Could you check a few things on this drawing? It's one solid part, dimensions in mm from its lowest x, y, z. A direction names the side the tool comes from. Round coordinates to 2 decimals unless told otherwise and drop trailing zeros. Loops run counter-clockwise (first coordinate to the right, second up) from the corner with the lowest first, then second, coordinate; pieces in that order, holes last. Notation, with made-up numbers: M 57.25,69.5 L 65.25,69.5 A32 ccw 65.25,104.5 Z; hole C -5,36 d10. An arc over 180 degrees is marked long. Write item = value, one per line. Start each with the question number.
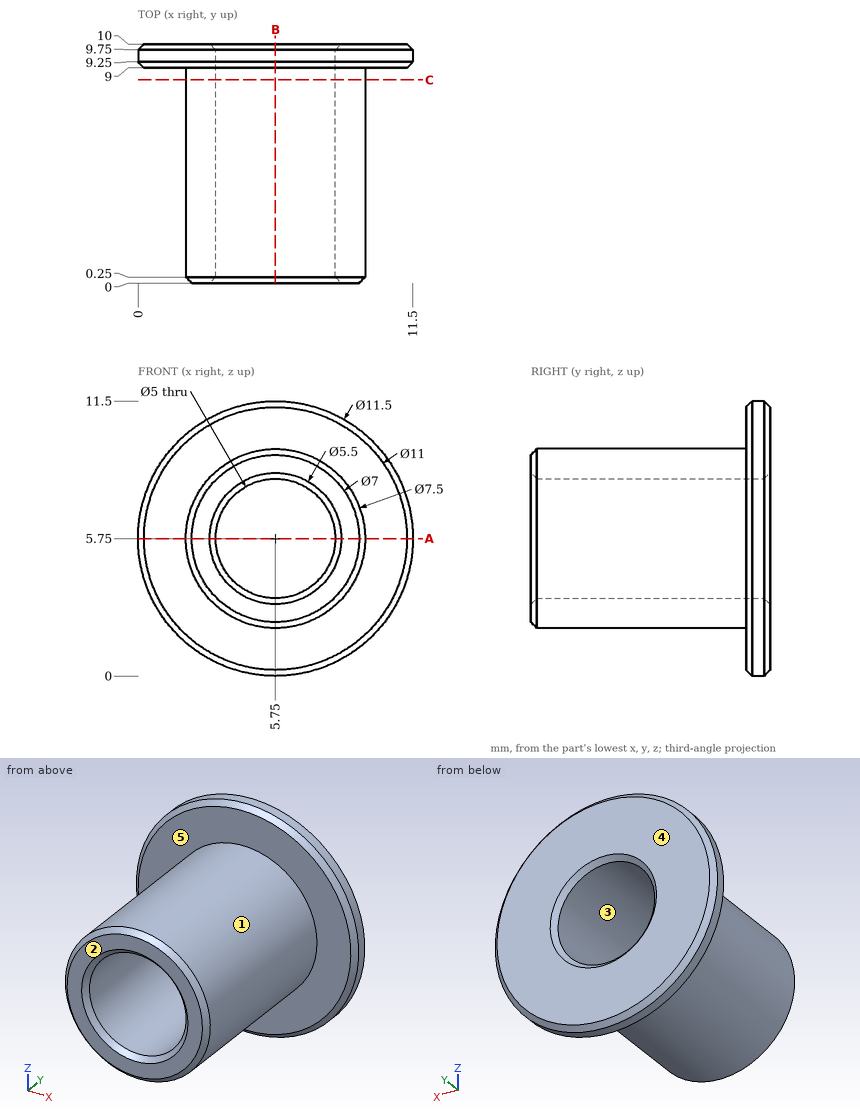
Item 1: I want a section at A-A, the plane z = 5.75. List the corners of the cut face in (x, y) for me.
Item 2: Please list where these lines run through material, in increasing order: line 1 (X direction, y = 7.5, z = 5.75); line 2 (Y direction, x = 2.5, z = 2.25). Write a range as [from, to].
Item 3: For the marked faces 4 and 5, which set-ups out of +Z, -Z, +X, -X, +Y, -Y let a thin tool reach every point of the face, with its end or its side?
Item 4: We'd pull the mould along Z, two halves only. Please class the marked faces 1, 2 and 3: released by +Z, released by -Z, zero draft, split by the parting line, or undercut.
Item 5: Will these pins go through, and if not, where does the flat tip stop? pin 1 Ø6 at (x, y) = (6.5, 4.5) entering from +Z; pin 2 Ø4 at (y, z) = (3, 5) entering from +X.
Item 6: I want a section at C-C, the plane y = 8.5. List the corners of the cut face in (x, z) for me.
Item 7: I want a section at B-B, the plane x = 5.75. List the corners of the cut face in (y, z) for me, then the cut area to 3 significant figures.
Worked out:
q1.outline = M 0,9.25 L 0.25,9 L 2,9 L 2,0.25 L 2.25,0 L 3,0 L 3.25,0.25 L 3.25,9.75 L 3,10 L 0.25,10 L 0,9.75 Z; M 8.25,0.25 L 8.5,0 L 9.25,0 L 9.5,0.25 L 9.5,9 L 11.25,9 L 11.5,9.25 L 11.5,9.75 L 11.25,10 L 8.5,10 L 8.25,9.75 Z
q2.line_1 = [2, 3.25], [8.25, 9.5]
q2.line_2 = [9, 10]
q3.face_4 = +Z, -Z, +X, -X, +Y
q3.face_5 = -Y
q4.face_1 = split by the parting line
q4.face_2 = zero draft
q4.face_3 = undercut
q5.pin_1 = 9.5
q5.pin_2 = 9.5
q6.outline = C 5.75,5.75 d7.5; hole C 5.75,5.75 d5
q7.outline = M 0,2.25 L 0.25,2 L 9,2 L 9,0.25 L 9.25,0 L 9.75,0 L 10,0.25 L 10,3 L 9.75,3.25 L 0.25,3.25 L 0,3 Z; M 0,8.5 L 0.25,8.25 L 9.75,8.25 L 10,8.5 L 10,11.25 L 9.75,11.5 L 9.25,11.5 L 9,11.25 L 9,9.5 L 0.25,9.5 L 0,9.25 Z
q7.area = 28.7 mm2
